from build123d import *

# Parameters (mm, degrees)
F0_W     = 50.8
F0_H     = 38.1
F1_DEPTH = 31.75
F2_W     = 25.4
F2_H     = 19.05
F3_DEPTH = 19.05
F4_DEPTH = 25.4
F6_DEPTH = 50.8


with BuildPart() as f1:
    # F0 (on Front) → F1 (new body)
    with BuildSketch(Plane.XZ):
        with Locations((-45.1402231145, 19.05)):
            Rectangle(F0_W, F0_H)
    extrude(amount=F1_DEPTH)

    # F2 (on face) → F3 (cut)
    with BuildSketch(Plane.XZ.offset(31.75)):
        with Locations((-45.1402231145, 28.575)):
            Rectangle(F2_W, F2_H)
    extrude(amount=-F3_DEPTH, mode=Mode.SUBTRACT)

    # F4 (cut): a face of the model
    f4_faces = [f1.faces().sort_by_distance(p)[0] for p in [
        (-45.1402231145, -12.7, 28.575),
    ]]
    extrude(f4_faces, amount=-F4_DEPTH, mode=Mode.SUBTRACT)

    # F5 (on face) → F6 (cut)
    with BuildSketch(Plane.YZ.offset(-19.7402231145)):
        with BuildLine():
            ThreePointArc((-31.75, 12.7), (-16.3850971413, 22.7350971413), (-6.35, 38.1))
            Line((-6.35, 38.1), (-31.75, 38.1))
            Line((-31.75, 38.1), (-31.75, 12.7))
        make_face()
    extrude(amount=-F6_DEPTH, mode=Mode.SUBTRACT)


solid = f1.part
Work out the finished part from the listing and answer in its coordinate system (mm). A direction names the side the tool comes from. Round coordinates to 2 decimals unless told otherwise and drop trailing zeros. Write each loop counter-clockwise with the first axis right and the second up, starting at its lowest first coordinate (ties: lowest second). Pieces come first, ordered by that corner, then holes. Notation, with made-up numbers: M 8,83.5 L 62,83.5 A13 ccw 62,89.5 Z; hole C -31.5,55 d11. An arc over 180 degrees is marked long. Use a Markdown table: item, result.
1) The part is cut by section D-D on z = 25. Give the vertices of the cut face in (x, y), plus the area to 3 significant figures.
Taken from the geometry:
| item | result |
|---|---|
| outline | M -70.54,-14.27 L -57.84,-14.27 L -57.84,0 L -70.54,0 Z; M -32.44,-14.27 L -19.74,-14.27 L -19.74,0 L -32.44,0 Z |
| area | 363 mm2 |
2) Which of the six approach directions +Z, -Z, +X, -X, +Y, -Y give full straight-line access (tool end or side, diameter ignored) to faces 5 (the face through (-32.44, -6, 26)), 6 (the face through (-45, -16, 0))?
Taken from the geometry:
| item | result |
|---|---|
| face 5 | +Z, +Y, -Y |
| face 6 | -Z, +X, -X, +Y, -Y |
3) The part is cut by section B-B on x = -37. Give the vertices of the cut face in (y, z), plus the area to 3 significant figures.
Taken from the geometry:
| item | result |
|---|---|
| outline | M -31.75,0 L 0,0 L 0,19.05 L -20.56,19.05 A44.68 cw -31.75,12.7 Z |
| area | 565 mm2 |
4) The part is cut by section A-A on z = 31. Give the vertices of the cut face in (x, y).
Taken from the geometry:
| item | result |
|---|---|
| outline | M -70.54,-9.87 L -57.84,-9.87 L -57.84,0 L -70.54,0 Z; M -32.44,-9.87 L -19.74,-9.87 L -19.74,0 L -32.44,0 Z |
5) The part is cut by section C-C on y = -2.5. Give the vertices of the cut face in (x, z).
Taken from the geometry:
| item | result |
|---|---|
| outline | M -70.54,0 L -19.74,0 L -19.74,38.1 L -32.44,38.1 L -32.44,19.05 L -57.84,19.05 L -57.84,38.1 L -70.54,38.1 Z |
6) Determine the mould class of faces 1 (the face through (-57.84, -6, 26)), 2 (the face through (-70.54, -12, 15)), 3 (the face through (-64, -3, 38.1)), 4 (the face through (-45, -10, 19.05)) for opening direction X: pulls with the +X half, pulls with the -X half, needs draft (parallel to the pull), parting line crosses it, or undercut.
Taken from the geometry:
| item | result |
|---|---|
| face 1 | undercut |
| face 2 | pulls with the -X half |
| face 3 | needs draft |
| face 4 | undercut |
7) Consider line 1 (X direction, y = -1, z = 23); line 2 (Z direction, x = -46.5, y = -12); line 3 (Y direction, x = -53.5, z = 14). Determine where each line is inside the solid, lowest interval first. Write a range as [from, to].
Taken from the geometry:
| item | result |
|---|---|
| line 1 | x = [-70.54, -57.84], [-32.44, -19.74] |
| line 2 | z = [0, 19.05] |
| line 3 | y = [-28.75, 0] |
8) Flat-ended cylindrical pins translate along their axes: pin 1 (4 mm diameter, centred on x = -36.5, z = 17, fed in from -Y); pin 2 (3 mm diameter, centred on x = -32.5, y = -4.5, fed in from +Z); pin 3 (16.5 mm diameter, centred on x = -45, y = -13, fed in from +Z); pin 4 (1.5 mm diameter, centred on x = -55.5, z = 30.5, fed in from +Y). Find the tip coordinate at first contact, or state that the pin passes through.
Taken from the geometry:
| item | result |
|---|---|
| pin 1 | stops at y = -26.78 |
| pin 2 | stops at z = 38.1 |
| pin 3 | stops at z = 19.05 |
| pin 4 | passes through |
